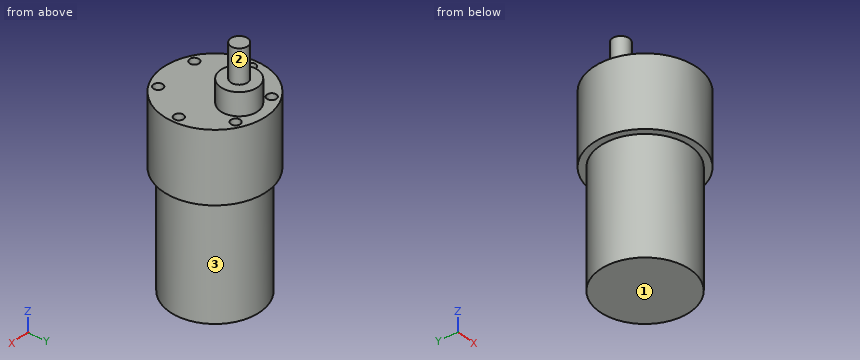
```python
from build123d import *

# Parameters (mm, degrees)
SKETCH1_R           = 18.4
BOSS_EXTRUDE1_DEPTH = 25
SKETCH2_R           = 16
BOSS_EXTRUDE2_DEPTH = 40.85
SKETCH3_R           = 1.675
CUT_EXTRUDE1_DEPTH  = 10
SKETCH4_R           = 6.55
BOSS_EXTRUDE3_DEPTH = 8
SKETCH5_R           = 3
BOSS_EXTRUDE4_DEPTH = 12


with BuildPart() as part:
    # Sketch1 → Boss-Extrude1 (new body)
    with BuildSketch(Plane.XY):
        Circle(SKETCH1_R)
    extrude(amount=-BOSS_EXTRUDE1_DEPTH)

    # Sketch2 → Boss-Extrude2 (add)
    with BuildSketch(Plane(origin=(0, 0, -25), x_dir=(-1, 0, 0), z_dir=(0, 0, -1))):
        Circle(SKETCH2_R)
    extrude(amount=BOSS_EXTRUDE2_DEPTH)

    # Sketch3 → Cut-Extrude1 (cut)
    with BuildSketch(Plane.XY):
        with Locations((15.65, 0)):
            Circle(SKETCH3_R)
        with Locations((7.825, -13.553297569)):
            Circle(SKETCH3_R)
        with Locations((-7.825, -13.553297569)):
            Circle(SKETCH3_R)
        with Locations((-15.65, 0)):
            Circle(SKETCH3_R)
        with Locations((-7.825, 13.553297569)):
            Circle(SKETCH3_R)
        with Locations((7.825, 13.553297569)):
            Circle(SKETCH3_R)
    extrude(amount=-CUT_EXTRUDE1_DEPTH, mode=Mode.SUBTRACT)

    # Sketch4 → Boss-Extrude3 (add)
    with BuildSketch(Plane.XY):
        with Locations((0, 8.5)):
            Circle(SKETCH4_R)
    extrude(amount=BOSS_EXTRUDE3_DEPTH)

    # Sketch5 → Boss-Extrude4 (add)
    with BuildSketch(Plane.XY.offset(8)):
        with Locations((0, 8.5)):
            Circle(SKETCH5_R)
    extrude(amount=BOSS_EXTRUDE4_DEPTH)


solid = part.part
```
Can you work these out from the model? Positions are in its coordinate system, mm. Face numbers are marked on the shaded views. A direction names the side the tool comes from. Coordinates: 2 decimals unless noted, no trailing zeros. Loops run counter-clockwise (first coordinate to the right, second up) from the corner with the lowest first, then second, coordinate; pieces in that order, holes last. Notation, with made-up numbers: M -36.75,52 L -17.75,52 A34 ccw -17.75,88 Z; hole C -20,69 d10. An arc over 180 degrees is marked long. Put each result on its own line as item: value. Start each with the question number.
(1) Imagine slicing it at D-D on z = -38. List the corners of the cut face in (x, y) for me, and give its area (3 significant figures).
(2) I need wall thicknesses on probe 1 along Z at (x, y) = (-4, -1); probe 2 along Z at (x, y) = (3.5, 11); probe 3 along Y at (x, z) = (15.65, -4.75) (3 decimals). Which ranges of each line are inside material? Lowest first, please.
(3) Which directions (+Z, -Z, +X, -X, +Y, -Y) give clear straight access to the entire face, cutting with the end or side of a thin tool? Please do the marked faces 1, 2 and 3.
(4) Will these pins go through, and if not, where does the flat tip stop? pin 1 Ø1.7 at (x, y) = (-8.5, -13.5) entering from +Z; pin 2 Ø2.5 at (x, y) = (16.5, 1) entering from +Z; pin 3 Ø1.5 at (x, z) = (1, -14.5) entering from -Y.
(5) Imagine slicing it at C-C on z = 4. List the corners of the cut face in (x, y) for me, and give its area (3 significant figures).
(6) Imagine slicing it at A-A on x = 0. List the corners of the cut face in (y, z) for me.
(7) Imagine slicing it at B-B on y = 0. List the corners of the cut face in (x, z) for me (3 decimals), and give its area (3 significant figures).
Worked answers:
1. outline: C 0,0 d32
1. area: 804 mm2
2. probe 1: z = -65.85 to 0
2. probe 2: z = -65.85 to 8
2. probe 3: y = -9.677 to -1.675, 1.675 to 9.677
3. face 1: -Z, +X, -X, +Y, -Y
3. face 2: +Z
3. face 3: -Z
4. pin 1: stops at z = -10
4. pin 2: stops at z = 0
4. pin 3: stops at y = -18.4
5. outline: C 0,8.5 d13.1
5. area: 135 mm2
6. outline: M -18.4,-25 L -16,-25 L -16,-65.85 L 16,-65.85 L 16,-25 L 18.4,-25 L 18.4,0 L 15.05,0 L 15.05,8 L 11.5,8 L 11.5,20 L 5.5,20 L 5.5,8 L 1.95,8 L 1.95,0 L -18.4,0 Z
7. outline: M -18.4,-25 L -16,-25 L -16,-65.85 L 16,-65.85 L 16,-25 L 18.4,-25 L 18.4,0 L 17.325,0 L 17.325,-10 L 13.975,-10 L 13.975,0 L -13.975,0 L -13.975,-10 L -17.325,-10 L -17.325,0 L -18.4,0 Z
7. area: 2,160 mm2
